Read the model definition and answer for the solid it produces. Units are mm, in the model's axes. Face numbers are marked on the shaded views. A direction names the side the tool comes from. Coordinates: 2 decimals unless noted, no trailing zeros. Order: outer loops, then holes, each group sorted by start corner. A loop starts at its lowest first (then second) coordinate and runs counter-clockwise, first axis right, second up. Notation, with made-up numbers: M 86,56 L 118,56 A23 ccw 118,69 Z; hole C -37,71.5 d5. An arc over 180 degrees is marked long. Use a Markdown table: item, result. Add a question column.
1) Find section D-D on y = 82.55. Write down the section's boundary in (x, z) (3 decimals), plus the area to 3 significant figures.
2) Each of these flat-tipped pins is pushed along its axis until it touches: pin 1 Ø5 at (x, y) = (-13, 52) entering from -Z; pin 2 Ø17.5 at (x, z) = (-17.5, 19.5) entering from +Y; pin 3 Ø5 at (x, z) = (1, 52.5) entering from -Y. Where does it stop, or does it pass through?
3) Find section A-A on z = 35. Count the separate pieces of the cut face and the enclosed holes in it, plus the area to 3 significant figures.
4) Find section C-C on y = 42.5. Write down the section's boundary in (x, z), plus the area to 3 significant figures.
5) The mould has two halves that part along Z. Classify the marked faces 4, 5 and 6: released by +Z, released by -Z, zero draft, split by the parting line, or undercut.
6) Find the intervals of material crossed by probe 1 along Z at (x, y) = (0, 5) (3 decimals); probe 2 along X at (y, z) = (65, 10) (3 decimals); probe 3 along X at (y, z) = (52.5, -8.5), in increasing order. Write a range as [from, to].
7) For the marked faces 1, 2 and 3, determine the directions among +Z, -Z, +X, -X, +Y, -Y from which every point of the face is accessible in a straight line to the end or side of a thin tool.
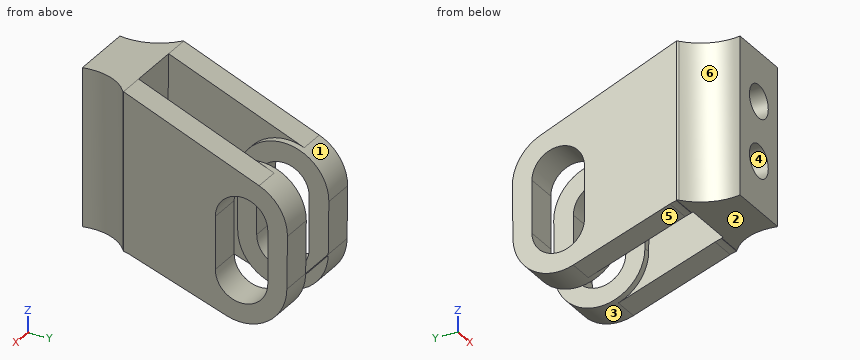
from build123d import *

# Parameters (mm, degrees)
BOSS_EXTRUDE1_DEPTH = 76.2
BOSS_EXTRUDE3_DEPTH = 25.4
SKETCH4_W           = 25.4
SKETCH4_H           = 94.262089718
CUT_EXTRUDE1_DEPTH  = 79.936326
BOSS_EXTRUDE4_START = 12.7
BOSS_EXTRUDE4_DEPTH = 3.175
BOSS_EXTRUDE5_START = -12.7
BOSS_EXTRUDE5_DEPTH = 3.175
SKETCH5_R           = 7.9375
CUT_EXTRUDE2_DEPTH  = 19.05


with BuildPart() as part:
    # Sketch2 → Boss-Extrude1 (new body)
    with BuildSketch(Plane.XY):
        with BuildLine():
            Line((-15.875, 0), (15.875, 0))
            ThreePointArc((15.875, 0), (16.884197435, 13.479245674), (24.665075731, 24.532140152))
            ThreePointArc((24.665075731, 24.532140152), (25.071711114, 24.932897242), (25.4, 25.4))
            Line((25.4, 25.4), (-25.4, 25.4))
            ThreePointArc((-25.4, 25.4), (-25.071711114, 24.932897242), (-24.665075731, 24.532140152))
            ThreePointArc((-24.665075731, 24.532140152), (-16.884197435, 13.479245674), (-15.875, 0))
        make_face()
    extrude(amount=BOSS_EXTRUDE1_DEPTH)

    # Sketch3 → Boss-Extrude3 (add, symmetric)
    with BuildSketch(Plane(origin=(0, 0, 0), x_dir=(0, 0, -1), z_dir=(1, 0, 0))):
        with BuildLine():
            Line((-28.575, 60.325), (-3.175, 60.627395043))
            ThreePointArc((-3.175, 60.627395043), (18.747604957, 82.55), (-3.175, 104.472604957))
            Line((-3.175, 104.472604957), (-28.575, 104.775))
            ThreePointArc((-28.575, 104.775), (-50.8, 82.55), (-28.575, 60.325))
        make_face()
        with BuildLine():
            ThreePointArc((-3.175, 69.85), (9.525, 82.55), (-3.175, 95.25))
            Line((-3.175, 95.25), (-28.575, 95.25))
            ThreePointArc((-28.575, 95.25), (-41.275, 82.55), (-28.575, 69.85))
            Line((-28.575, 69.85), (-3.175, 69.85))
        make_face(mode=Mode.SUBTRACT)
        with BuildLine():
            Line((-76.2, 25.4), (0.270677579, 25.353877505))
            ThreePointArc((0.270677579, 25.353877505), (0.607218741, 26.92535435), (1.075018311, 28.462872802))
            Line((1.075018311, 28.462872802), (17.510481505, 75.289733957))
            ThreePointArc((17.510481505, 75.289733957), (9.502473403, 64.664746962), (-3.175, 60.627395043))
            Line((-3.175, 60.627395043), (-28.575, 60.325))
            ThreePointArc((-28.575, 60.325), (-47.046096671, 70.190015665), (-49.119653814, 91.02748929))
            Line((-49.119653814, 91.02748929), (-76.2, 25.4))
        make_face()
    extrude(amount=BOSS_EXTRUDE3_DEPTH, both=True)

    # Sketch4 → Cut-Extrude1 (cut)
    with BuildSketch(Plane(origin=(0, 104.420005444, -1.243153229), x_dir=(1, 0, 0), z_dir=(0, 0.999929139, -0.011904473))):
        with Locations((0, -29.365929167)):
            Rectangle(SKETCH4_W, SKETCH4_H)
    extrude(amount=-CUT_EXTRUDE1_DEPTH, mode=Mode.SUBTRACT)

    # Sketch3<7> → Boss-Extrude4 (add)
    with BuildSketch(Plane(origin=(0, 0, 0), x_dir=(0, 0, -1), z_dir=(1, 0, 0)).offset(BOSS_EXTRUDE4_START)):
        with BuildLine():
            Line((-28.575, 60.325), (-3.175, 60.627395043))
            ThreePointArc((-3.175, 60.627395043), (18.747604957, 82.55), (-3.175, 104.472604957))
            Line((-3.175, 104.472604957), (-28.575, 104.775))
            ThreePointArc((-28.575, 104.775), (-50.8, 82.55), (-28.575, 60.325))
        make_face()
        with BuildLine():
            ThreePointArc((-3.175, 69.85), (9.525, 82.55), (-3.175, 95.25))
            Line((-3.175, 95.25), (-28.575, 95.25))
            ThreePointArc((-28.575, 95.25), (-41.275, 82.55), (-28.575, 69.85))
            Line((-28.575, 69.85), (-3.175, 69.85))
        make_face(mode=Mode.SUBTRACT)
    extrude(amount=-BOSS_EXTRUDE4_DEPTH)

    # Sketch3<8> → Boss-Extrude5 (add)
    with BuildSketch(Plane(origin=(0, 0, 0), x_dir=(0, 0, -1), z_dir=(1, 0, 0)).offset(BOSS_EXTRUDE5_START)):
        with BuildLine():
            Line((-28.575, 60.325), (-3.175, 60.627395043))
            ThreePointArc((-3.175, 60.627395043), (18.747604957, 82.55), (-3.175, 104.472604957))
            Line((-3.175, 104.472604957), (-28.575, 104.775))
            ThreePointArc((-28.575, 104.775), (-50.8, 82.55), (-28.575, 60.325))
        make_face()
        with BuildLine():
            ThreePointArc((-3.175, 69.85), (9.525, 82.55), (-3.175, 95.25))
            Line((-3.175, 95.25), (-28.575, 95.25))
            ThreePointArc((-28.575, 95.25), (-41.275, 82.55), (-28.575, 69.85))
            Line((-28.575, 69.85), (-3.175, 69.85))
        make_face(mode=Mode.SUBTRACT)
    extrude(amount=BOSS_EXTRUDE5_DEPTH)

    # Sketch5 → Cut-Extrude2 (cut)
    with BuildSketch(Plane.XZ):
        with Locations((0, 52.3875)):
            Circle(SKETCH5_R)
        with Locations((0, 23.8125)):
            Circle(SKETCH5_R)
    extrude(amount=-CUT_EXTRUDE2_DEPTH, mode=Mode.SUBTRACT)


solid = part.part
Check result:
| question | item | result |
|---|---|---|
| 1 | outline | M -25.4,-18.748 L -9.525,-18.748 L -9.525,-9.525 L -25.4,-9.525 Z; M -25.4,41.275 L -9.525,41.275 L -9.525,50.8 L -12.7,50.8 L -12.7,52.618 L -25.4,52.618 Z; M 9.525,-18.748 L 25.4,-18.748 L 25.4,-9.525 L 9.525,-9.525 Z; M 9.525,41.275 L 25.4,41.275 L 25.4,52.618 L 12.7,52.618 L 12.7,50.8 L 9.525,50.8 Z |
| 1 | area | 641 mm2 |
| 2 | pin 1 | stops at z = -10.21 |
| 2 | pin 2 | stops at y = 104.77 |
| 2 | pin 3 | stops at y = 19.05 |
| 3 | separate pieces | 3 |
| 3 | enclosed holes | 0 |
| 3 | area | 2,470 mm2 |
| 4 | outline | M -25.4,-6 L -12.7,-6 L -12.7,69.14 L -25.4,69.14 Z; M 12.7,-6 L 25.4,-6 L 25.4,69.14 L 12.7,69.14 Z |
| 4 | area | 1,910 mm2 |
| 5 | face 4 | undercut |
| 5 | face 5 | released by -Z |
| 5 | face 6 | zero draft |
| 6 | probe 1 | z = [0, 15.875], [31.75, 44.45], [60.325, 76.2] |
| 6 | probe 2 | x = [-25.4, -9.525], [9.525, 25.4] |
| 6 | probe 3 | x = [-25.4, -12.7], [12.7, 25.4] |
| 7 | face 1 | +Z |
| 7 | face 2 | -Z, +X, -X, -Y |
| 7 | face 3 | -Z |
